```python
from build123d import *


with BuildPart() as part:
    # Sketch1 → Revolve1 (revolve)
    with BuildSketch(Plane.XY, mode=Mode.PRIVATE) as revolve1_sk:
        with BuildLine():
            Line((15.446351252, 33.000061), (15.446351252, 57.15))
            Line((15.446351252, 57.15), (33.226351252, 57.15))
            Line((33.226351252, 57.15), (33.226351252, 59.69))
            Line((33.226351252, 59.69), (12.906351252, 59.69))
            Line((12.906351252, 59.69), (12.906351252, 33.579511809))
            ThreePointArc((12.906351252, 33.579511809), (7.576431779, 27.783815658), (0, 25.64003))
            add(Edge.make_bspline(
                [(-43.66006, 46.20006), (-43.66006, 45.606103818), (-43.544794528, 44.432570076), (-42.839776678, 42.039054169), (-41.001665327, 38.971251765), (-37.14971819, 35.345133748), (-31.752396376, 32.048371643), (-25.035415413, 29.287682921), (-17.281065772, 27.214070609), (-8.82958884, 25.929831174), (-2.92413983, 25.64003), (0, 25.64003)],
                knots=[3.141592654, 3.141592654, 3.141592654, 3.141592654, 3.239767424, 3.337942194, 3.534291735, 3.730641276, 3.926990817, 4.123340358, 4.319689899, 4.51603944, 4.71238898, 4.71238898, 4.71238898, 4.71238898], degree=3))
            ThreePointArc((-43.66006, 46.20006), (-44.93006, 47.47006), (-46.20006, 46.20006))
            add(Edge.make_bspline(
                [(-46.20006, 46.20006), (-46.20006, 23.10003), (0, 23.10003)],
                knots=[3.141592654, 3.141592654, 3.141592654, 4.71238898, 4.71238898, 4.71238898], degree=2, weights=[1, 0.707106781, 1]))
            ThreePointArc((0, 23.10003), (9.1733361, 25.787457832), (15.446351252, 33.000061))
        make_face()
    revolve(revolve1_sk.sketch.rotate(Axis((0, 0, 0), (1, 0, 0)), 90), axis=Axis((0, 0, 0), (1, 0, 0)))


solid = part.part
```
Work out the finished part from the listing and answer in its coordinate system (mm). A direction names the side the tool comes from. Give positions to 0.01 mm unless a question says otherwise; leave off trailing zeros. Write each loop counter-clockwise with the first axis right and the second up, starting at its lowest first coordinate (ties: lowest second). Pieces come first, ordered by that corner, then holes.
(1) The mould has two halves that part along Z. Classify faces 3 (the cylindrical face through (22.924, -17.929, 56.934)), 4 (the flat face through (12.906, 26, 26)), 5 (the cylindrical face through (24.461, -2.513, -57.095)): pulls with the +Z half, pulls with the -Z half, needs draft (parallel to the pull), parting line crosses it, or undercut.
Final values:
face 3: parting line crosses it
face 4: needs draft
face 5: undercut
(2) Which of the six approach directions +Z, -Z, +X, -X, +Y, -Y give full straight-line access (tool end or side, diameter ignored) to faces 1 (the flat face through (15.446, 25, -25)), 2 (the flat face through (33.226, 30.7, -48.4))?
Final values:
face 1: +X
face 2: +Z, -Z, +X, +Y, -Y
(3) The part is cut by section A-A on y = -49. Write down the section's boundary in (x, z).
Final values:
outline: (12.91, -34.09) - (33.23, -34.09) - (33.23, -29.41) - (15.45, -29.41) - (15.45, 29.41) - (33.23, 29.41) - (33.23, 34.09) - (12.91, 34.09) - close
(4) Straight lines are drawn through the part: line 1 (Y direction, x = 26, z = 0); line 2 (X direction, y = -47, z = 14.5); line 3 (Y direction, x = 20, z = 44.5). For each, find the intervals that lie inside material, in ascending order.
Final values:
line 1: y = -59.69 to -57.15, 57.15 to 59.69
line 2: x = 12.91 to 15.45
line 3: y = -39.78 to -35.86, 35.86 to 39.78
(5) The part is cut by section D-D on x = 7. Write down the section's boundary in (y, z).
Final values:
outline: circle Ø54.89 at (0, 0); hole circle Ø49.22 at (0, 0)
(6) The part is cut by section C-C on y = 52.5. Write down the section's boundary in (x, z), plus the area to 3 significant figures.
Final values:
outline: (12.91, -28.4) - (33.23, -28.4) - (33.23, -22.58) - (15.45, -22.58) - (15.45, 22.58) - (33.23, 22.58) - (33.23, 28.4) - (12.91, 28.4) - close
area: 351 mm2
(7) The part is cut by section B-B on x = 20. Write down the section's boundary in (y, z), plus the area to 3 significant figures.
Final values:
outline: circle Ø119.38 at (0, 0); hole circle Ø114.3 at (0, 0)
area: 932 mm2
(8) Flat-ended cylindrical pins translate along their axes: pin 1 Ø2 at (x, z) = (15, 14) entering from -Y; pin 2 Ø4 at (x, z) = (-26.5, 23.5) entering from -Y; pin 3 Ø1.5 at (x, z) = (-37.5, 23.5) entering from -Y; pin 4 Ø1 at (y, z) = (-2, -21) entering from +X. Find the tip coordinate at first contact, or state that the pin passes through.
Final values:
pin 1: stops at y = -58.26
pin 2: stops at y = -21.16
pin 3: stops at y = -28.12
pin 4: passes through
